Can you work these out from the model? Positions are in its coordinate system, mm. A direction names the side the tool comes from. Give positions to 0.01 mm unless a question says otherwise; leave off trailing zeros. Loops run counter-clockwise (first coordinate to the right, second up) from the corner with the lowest first, then second, coordinate; pieces in that order, holes last. Notation, with made-up numbers: M 2,59.25 L 48,59.25 A30 cw 48,89.25 Z; hole C -22.75,-30 d4. An arc over 180 degrees is marked long. Use CSV: the item, a comma, the result in double quotes.
from build123d import *

# Parameters (mm, degrees)
SKETCH2_W           = 25.4
SKETCH2_H           = 50.8
SKETCH2_R           = 6.35
BOSS_EXTRUDE1_DEPTH = 12.7
BOSS_EXTRUDE2_DEPTH = 6.35


with BuildPart() as part:
    # Sketch2 → Boss-Extrude1 (new body)
    with BuildSketch(Plane.XY):
        with Locations((0, -61.205719116)):
            Rectangle(SKETCH2_W, SKETCH2_H)
        with Locations((0, -61.205719116)):
            Circle(SKETCH2_R, mode=Mode.SUBTRACT)
    extrude(amount=-BOSS_EXTRUDE1_DEPTH)

    # Sketch3 → Boss-Extrude2 (add)
    with BuildSketch(Plane.XY):
        with BuildLine():
            Line((-57.15, -45.330719116), (57.15, -45.330719116))
            ThreePointArc((57.15, -45.330719116), (73.025, -61.205719116), (57.15, -77.080719116))
            Line((57.15, -77.080719116), (-57.15, -77.080719116))
            ThreePointArc((-57.15, -77.080719116), (-73.025, -61.205719116), (-57.15, -45.330719116))
        make_face()
        with BuildLine():
            Line((-57.15, -58.030719116), (57.15, -58.030719116))
            ThreePointArc((57.15, -58.030719116), (60.325, -61.205719116), (57.15, -64.380719116))
            Line((57.15, -64.380719116), (-57.15, -64.380719116))
            ThreePointArc((-57.15, -64.380719116), (-60.325, -61.205719116), (-57.15, -58.030719116))
        make_face(mode=Mode.SUBTRACT)
    extrude(amount=BOSS_EXTRUDE2_DEPTH)


solid = part.part
Q1. I'm going to push flat-ended pins straight in: P1, Ø10, axis at y = -68, z = -9.5, coming from the +X side; P2, Ø4, axis at x = -56, z = 2, coming from the -Y side; P3, Ø7.5, axis at x = 0, y = -61.21, coming from the -Z side. Where does each tip first touch, or does it pass through?
Model answer:
P1,"x = 12.7"
P2,"y = -77.08"
P3,"z = 0"
Q2. I want a section at C-C, the plane x = 0. Please give me the cut outline in (y, z).
Model answer:
outline,"M -86.61,-12.7 L -67.56,-12.7 L -67.56,0 L -64.38,0 L -64.38,6.35 L -77.08,6.35 L -77.08,0 L -86.61,0 Z; M -58.03,0 L -54.86,0 L -54.86,-12.7 L -35.81,-12.7 L -35.81,0 L -45.33,0 L -45.33,6.35 L -58.03,6.35 Z"
Q3. I want a section at A-A, the plane x = 29.5. Please give me the cut outline in (y, z).
Model answer:
outline,"M -77.08,0 L -64.38,0 L -64.38,6.35 L -77.08,6.35 Z; M -58.03,0 L -45.33,0 L -45.33,6.35 L -58.03,6.35 Z"
Q4. I want a section at B-B, the plane z = 3.75. Please give me the cut outline in (x, y) (3 decimals).
Model answer:
outline,"M -57.15,-77.081 L 57.15,-77.081 A15.875 ccw 57.15,-45.331 L -57.15,-45.331 A15.875 ccw Z; hole M -57.15,-64.381 L 57.15,-64.381 A3.175 ccw 57.15,-58.031 L -57.15,-58.031 A3.175 ccw Z"
Q5. I want a section at D-D, the plane y = -80. Please give me the cut outline in (x, z).
Model answer:
outline,"M -12.7,-12.7 L 12.7,-12.7 L 12.7,0 L -12.7,0 Z"
Q6. For faces 1 (the flat face through (9, -61, 0)), 2 (the flat face through (0, -82, 0)), 3 (the cylindrical face through (-60.324, -61.276, 3.131)), which set-ups out of +Z, -Z, +X, -X, +Y, -Y let a thin tool reach every point of the face, with its end or its side?
Model answer:
face 1,"+Z"
face 2,"+Z, +X, -X, -Y"
face 3,"+Z, -Z"
Q7. If we mould it in two halves opening along Y, with no side actions, what happens to faces 4 (the flat face through (1, -64.381, 3)), 5 (the flat face through (-42, -65, 0)), 6 (the flat face through (0, -86.606, -6))? For each: released by +Y, released by -Y, zero draft, split by the parting line, or undercut.
Model answer:
face 4,"undercut"
face 5,"zero draft"
face 6,"released by -Y"
Q8. Please list where these lines run through material, in increasing order: L1, parallel to Y at x = -28, z = 4.25; L2, parallel to Y at x = 0, z = -6; L3, parallel to X at y = -79.5, z = -8.75. Write a range as from..to.
Model answer:
L1,"-77.08..-64.38, -58.03..-45.33"
L2,"-86.61..-67.56, -54.86..-35.81"
L3,"-12.7..12.7"
